Part model, mm, in its own coordinate system. Face numbers are marked on the shaded views. A direction names the side the tool comes from. Coordinates: 2 decimals unless noted, no trailing zeros. Write each loop counter-clockwise with the first axis right and the second up, starting at its lowest first coordinate (ties: lowest second). Pieces come first, ordered by that corner, then holes. Notation, with made-up numbers: M 8,-6 L 29,-6 A21 ccw 29,25 Z; hole C 49.5,-19.75 d1. An arc over 180 degrees is marked long. Use a Markdown table: item, result. Add a question column.
Q1. Slice it at B-B on x = 0. Write the cut outline in (y, z) (3 decimals), then the cut area to 3 significant figures.
Q2. Wall check: L1, parallel to X at y = 14, z = 0; L2, parallel to Y at x = -45.5, z = 20; L3, parallel to Z at x = -2.5, y = 8. Give the ranges that are in metal, low to high. Write a range as from..to.
Q3. Mould opens along X. For the marked faces 3, 4 and 5 say: released by +X, released by -X, zero draft, split by the parting line, or undercut.
Q4. Slice it at A-A on z = 0. Write the cut outline in (x, y) (3 decimals), then the cut area to 3 significant figures.
Q5. Tool access for the marked faces 1 and 2: list every direction of +Z, -Z, +X, -X, +Y, -Y with a clear straight run to the whole face (end or side of a thin tool).
Q6. Pin check, flat tips, straight feed: pin 1 Ø3 at (y, z) = (1.5, 1) entering from -X; pin 2 Ø8 at (x, y) = (39.5, 21) entering from -Z; pin 3 Ø6 at (y, z) = (8.5, -5) entering from +X; pin 4 Ø1.5 at (x, z) = (-11.5, -30.5) entering from +Y. Stop position of each tip, or through.
Q7. Slice it at C-C on y = 16.5. Write the cut outline in (x, z), then the cut area to 3 significant figures.
from build123d import *

# Parameters (mm, degrees)
SKETCH1_R           = 50.8
SKETCH1_R_2         = 34.798
BOSS_EXTRUDE1_DEPTH = 12.7
SKETCH2_R           = 45.72
SKETCH2_R_2         = 34.798
BOSS_EXTRUDE2_DEPTH = 12.7
FILLET1_R           = 5.588
SKETCH3_W           = 12.7
SKETCH3_H           = 12.7
CUT_EXTRUDE1_DEPTH  = 6.35
CIRPATTERN1_COUNT   = 4


with BuildPart() as part:
    # Sketch1 → Boss-Extrude1 (new body)
    with BuildSketch(Plane(origin=(0, 0, 0), x_dir=(1, 0, 0), z_dir=(0, 1, 0))):
        with Locations(Location((0, 0, 0), (0, 0, 270))):
            Circle(SKETCH1_R)
        with Locations(Location((0, 0, 0), (0, 0, 270))):
            Circle(SKETCH1_R_2, mode=Mode.SUBTRACT)
    extrude(amount=BOSS_EXTRUDE1_DEPTH)

    # Sketch2 → Boss-Extrude2 (add)
    with BuildSketch(Plane(origin=(0, 12.7, 0), x_dir=(1, 0, 0), z_dir=(0, 1, 0))):
        with Locations(Location((0, 0, 0), (0, 0, 270))):
            Circle(SKETCH2_R)
        with Locations(Location((0, 0, 0), (0, 0, 270))):
            Circle(SKETCH2_R_2, mode=Mode.SUBTRACT)
    extrude(amount=BOSS_EXTRUDE2_DEPTH)

    # Fillet1
    fillet1_edges = [part.edges().sort_by_distance(p)[0] for p in [
        (0, 0, -34.798),
    ]]
    fillet(fillet1_edges, radius=FILLET1_R)

    # Sketch3 → Cut-Extrude1 (cut)
    with BuildSketch(Plane.XZ):
        with Locations((34.925, 0)):
            Rectangle(SKETCH3_W, SKETCH3_H)
    cut_extrude1 = extrude(amount=-CUT_EXTRUDE1_DEPTH, mode=Mode.SUBTRACT)

    # CirPattern1: Cut-Extrude1 ×4 about axis
    cirpattern1_axis = Axis((0, 0, 0), (0, 1, 0))
    for i in range(1, CIRPATTERN1_COUNT):
        add(cut_extrude1.rotate(cirpattern1_axis, i * 360 / CIRPATTERN1_COUNT), mode=Mode.SUBTRACT)


solid = part.part
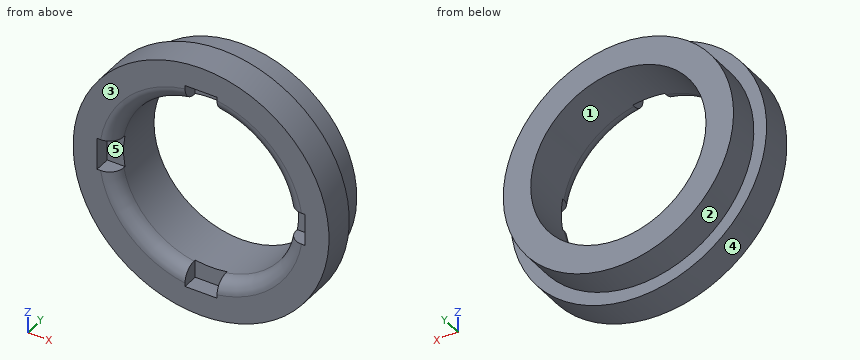
Recorded:
| question | item | result |
|---|---|---|
| 1 | outline | M 0,-50.8 L 12.7,-50.8 L 12.7,-45.72 L 25.4,-45.72 L 25.4,-34.798 L 6.35,-34.798 L 6.35,-41.275 L 0,-41.275 Z; M 0,41.275 L 6.35,41.275 L 6.35,34.798 L 25.4,34.798 L 25.4,45.72 L 12.7,45.72 L 12.7,50.8 L 0,50.8 Z |
| 1 | area | 602 mm² |
| 2 | L1 | -45.72..-34.8, 34.8..45.72 |
| 2 | L2 | 0..12.7 |
| 2 | L3 | -50.74..-34.71, 34.71..50.74 |
| 3 | face 3 | zero draft |
| 3 | face 4 | split by the parting line |
| 3 | face 5 | undercut |
| 4 | outline | M -50.8,0 L -41.275,0 L -41.275,6.35 L -34.798,6.35 L -34.798,25.4 L -45.72,25.4 L -45.72,12.7 L -50.8,12.7 Z; M 34.798,6.35 L 41.275,6.35 L 41.275,0 L 50.8,0 L 50.8,12.7 L 45.72,12.7 L 45.72,25.4 L 34.798,25.4 Z |
| 4 | area | 602 mm² |
| 5 | face 1 | +Y, -Y |
| 5 | face 2 | +Y |
| 6 | pin 1 | x = -50.8 |
| 6 | pin 2 | z = -28.81 |
| 6 | pin 3 | x = 50.76 |
| 6 | pin 4 | through |
| 7 | outline | C 0,0 d91.44; hole C 0,0 d69.6 |
| 7 | area | 2,760 mm² |
